Model file for the job. Use its own axes, mm. A direction names the side the tool comes from. Coordinates: 2 decimals unless noted, no trailing zeros. Write each loop counter-clockwise with the first axis right and the second up, starting at its lowest first coordinate (ties: lowest second). Pieces come first, ordered by that corner, then holes.
Q1. Band-saw the part on B-B, the plane y = 0.6. Write the cut outline in (x, z), plus the area to 3 significant figures.
Q2. Band-saw the part on A-A, the plane x = 6. Write the cut outline in (y, z), plus the area to 3 significant figures.
Q3. Band-saw the part on D-D, the plane z = -7.5. Write the cut outline in (x, y).
Q4. Which spindle directions (+Z, -Z, +X, -X, +Y, -Y) get a long thin tool onto all of the face, cutting with end or side? Do faces 5 (the flat face through (5, 2, -2.629)), 6 (the flat face through (8, 2, 15.456)), 7 (the flat face through (5, 2, -9.972)). Say none if no direction does.
Q5. Drill centre lines: probe 1 along Z at (x, y) = (6, 1.7); probe 2 along Y at (x, z) = (10.75, -7); probe 3 along X at (y, z) = (1.1, 10). Where is each one in solid material? Low to high.
Q6. Pin check, flat tips, straight feed: P1, Ø2, axis at x = 12.5, z = 5, coming from the +Y side; P2, Ø0.8, axis at x = 7, y = 1.5, coming from the -Z side; P3, Ø0.8, axis at y = 2, z = 12, coming from the -X side. Stop position of each tip, or through.
Q7. Pull direction Z, two halves, no side cores. Call faces 1 (the flat face through (4.8, 0.5, -15.264)), 2 (the cylindrical face through (-8.771, 1.74, -14.076)), 3 (the flat face through (5, 2, -6.369)), 4 (the flat face through (2.874, 2, -8)): released by +Z, released by -Z, zero draft, split by the parting line, or undercut.
Q8. Band-saw the part on C-C, the plane z = 7.5. Write the cut outline in (x, y).
from build123d import *

# Parameters (mm, degrees)
BOSS_EXTRUDE1_DEPTH = 1
SKETCH2_W           = 4.317372505
SKETCH2_H           = 3.603476264
SKETCH2_H_2         = 3.297520732
SKETCH2_W_2         = 5.830152634
SKETCH2_H_3         = 12.102241037
BOSS_EXTRUDE2_DEPTH = 1.5
SKETCH3_R           = 1.433043964
SKETCH3_R_2         = 1.189827068
BOSS_EXTRUDE3_DEPTH = 1.5


with BuildPart() as part:
    # Sketch1 → Boss-Extrude1 (new body)
    with BuildSketch(Plane(origin=(0, 0, 0), x_dir=(1, 0, 0), z_dir=(0, 1, 0))):
        with BuildLine():
            Line((-6.992736077, 15.263922518), (17.007263923, 15.263922518))
            Line((17.007263923, 15.263922518), (17.007263923, -16.736077482))
            Line((17.007263923, -16.736077482), (-6.992736077, -16.736077482))
            ThreePointArc((-6.992736077, -16.736077482), (-11.235376765, -14.978718169), (-12.992736077, -10.736077482))
            Line((-12.992736077, -10.736077482), (-12.992736077, 9.263922518))
            ThreePointArc((-12.992736077, 9.263922518), (-11.235376765, 13.506563205), (-6.992736077, 15.263922518))
        make_face()
    extrude(amount=BOSS_EXTRUDE1_DEPTH)

    # Sketch2 → Boss-Extrude2 (add)
    with BuildSketch(Plane(origin=(0, 1, 0), x_dir=(1, 0, 0), z_dir=(0, 1, 0))):
        with Locations((5.032824182, 8.170628001)):
            Rectangle(SKETCH2_W, SKETCH2_H)
        with Locations((5.032824182, 4.278193734)):
            Rectangle(SKETCH2_W, SKETCH2_H_2)
        with Locations((7.947900499, -9.404817551)):
            Rectangle(SKETCH2_W_2, SKETCH2_H_3)
    extrude(amount=BOSS_EXTRUDE2_DEPTH)

    # Sketch3 → Boss-Extrude3 (add)
    with BuildSketch(Plane(origin=(0, 1, 0), x_dir=(1, 0, 0), z_dir=(0, 1, 0))):
        with Locations((-8.616192044, -13.076283933)):
            Circle(SKETCH3_R)
        with Locations((-8.616192044, 12.895941215)):
            Circle(SKETCH3_R_2)
    extrude(amount=BOSS_EXTRUDE3_DEPTH)


solid = part.part
Answer sheet:
1. outline: (-12.99, -9.26) arc R6 ccw to (-6.99, -15.26) - (17.01, -15.26) - (17.01, 16.74) - (-6.99, 16.74) arc R6 ccw to (-12.99, 10.74) - close
1. area: 945 mm2
2. outline: (0, -15.26) - (1, -15.26) - (1, -9.97) - (2.5, -9.97) - (2.5, -6.37) - (1, -6.37) - (1, -5.93) - (2.5, -5.93) - (2.5, -2.63) - (1, -2.63) - (1, 3.35) - (2.5, 3.35) - (2.5, 15.46) - (1, 15.46) - (1, 16.74) - (0, 16.74) - close
2. area: 60.5 mm2
3. outline: (-12.99, 0) - (17.01, 0) - (17.01, 1) - (7.19, 1) - (7.19, 2.5) - (2.87, 2.5) - (2.87, 1) - (-12.99, 1) - close
4. face 5: +X, -X, +Y
4. face 6: +Z, +X, -X, +Y
4. face 7: -Z, +X, -X, +Y
5. probe 1: z = -9.97 to -6.37, -5.93 to -2.63, 3.35 to 15.46
5. probe 2: y = 0 to 1
5. probe 3: x = 5.03 to 10.86
6. P1: stops at y = 1
6. P2: stops at z = -9.97
6. P3: stops at x = -9.88
7. face 1: released by -Z
7. face 2: undercut
7. face 3: undercut
7. face 4: zero draft
8. outline: (-12.99, 0) - (17.01, 0) - (17.01, 1) - (10.86, 1) - (10.86, 2.5) - (5.03, 2.5) - (5.03, 1) - (-12.99, 1) - close
